Part print with two shaded views. Sizes in mm from the minimum x, y, z corner. A direction names the side the tool comes from. Give positions to 0.01 mm unless a question says otherwise; leave off trailing zeros. Order: outer loops, then holes, each group sorted by start corner. A loop starts at its lowest first (then second) coordinate and runs counter-clockwise, first axis right, second up. Notation, with made-up numbers: (73.5, -18) -> (109.5, -18) arc R6 ccw to (109.5, -8) -> close; hole circle Ø7 at (38.25, -21.5). An arc over 180 degrees is marked (long way). Answer as CSV lines item,"result".
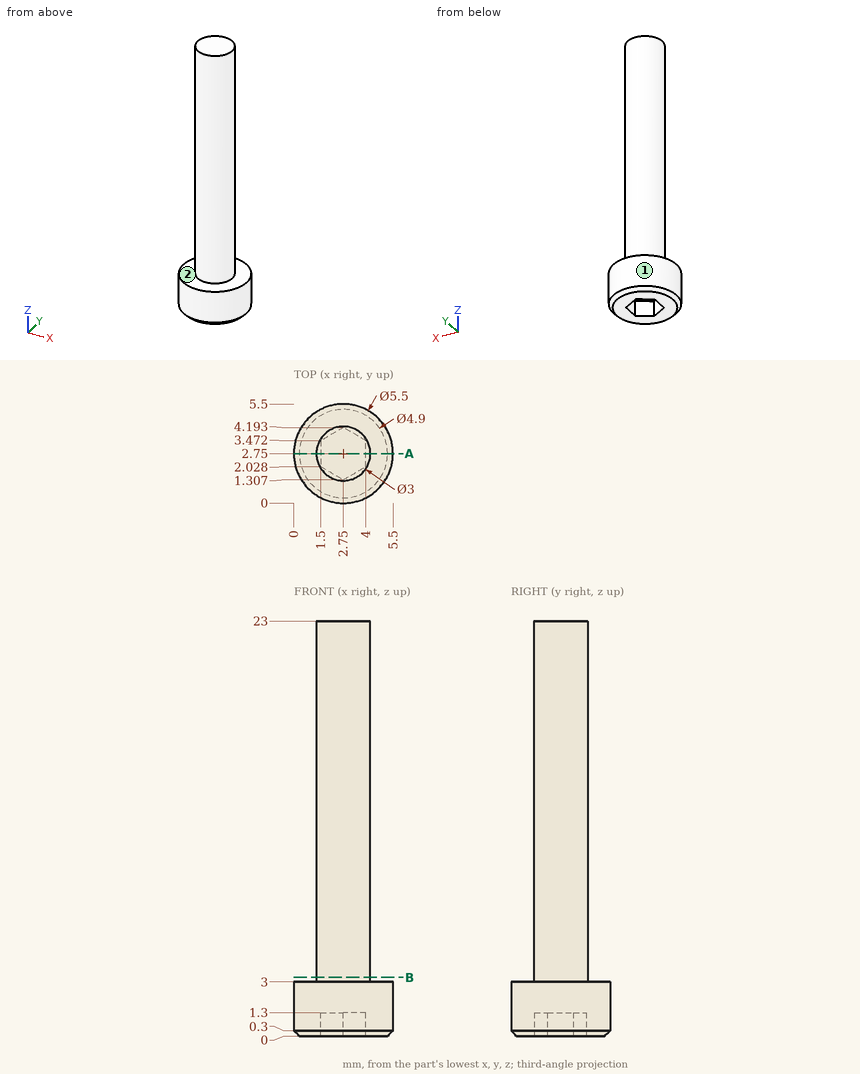
1) Pin check, flat tip, straight feed: P1, Ø3, axis at y = 3, z = 5.5, coming from the +X side. Stop position of the tip, or through.
Data:
P1,"stops at x = 4.25"
2) Wall check: line 1 along Z through (x, y) = (4.75, 2.3); line 2 along X through (y, z) = (2, 8.25); line 3 along X through (y, z) = (2.5, 11.5). Give the ranges that are in metal, low to high. Write a range as [from, to].
Data:
line 1,"z = [0, 3]"
line 2,"x = [1.45, 4.05]"
line 3,"x = [1.27, 4.23]"
3) Band-saw the part on A-A, the plane y = 2.75. Write the cut outline in (x, z).
Data:
outline,"(0, 0.3) -> (0.3, 0) -> (1.5, 0) -> (1.5, 1.3) -> (4, 1.3) -> (4, 0) -> (5.2, 0) -> (5.5, 0.3) -> (5.5, 3) -> (4.25, 3) -> (4.25, 23) -> (1.25, 23) -> (1.25, 3) -> (0, 3) -> close"
4) Band-saw the part on B-B, the plane z = 3.25. Write the cut outline in (x, y).
Data:
outline,"circle Ø3 at (2.75, 2.75)"
5) Which spindle directions (+Z, -Z, +X, -X, +Y, -Y) get a long thin tool onto all of the face, cutting with end or side? Do the marked faces 1 and 2. Say none if no direction does.
Data:
face 1,"+Z, -Z"
face 2,"+Z"
